Part model, mm, in its own coordinate system. A direction names the side the tool comes from. Coordinates: 2 decimals unless noted, no trailing zeros. Write each loop counter-clockwise with the first axis right and the second up, starting at its lowest first coordinate (ties: lowest second). Pieces come first, ordered by that corner, then holes. Notation, with made-up numbers: (37.5, 29) -> (69.5, 29) arc R31 cw to (69.5, 68) -> close; hole circle Ø11 at (71.25, -27). An arc over 180 degrees is marked (long way). Write item = value, one per line. Start each with the question number.
Q1. Band-saw the part on B-B, the plane x = -5. Give the number of separate pieces and of enclosed holes in the cut face, plus the area to 3 significant figures.
Q2. Band-saw the part on A-A, the plane z = 2.5. List the corners of the cut face in (x, y), plus the area to 3 significant figures.
Q3. Pin check, flat tips, straight feed: P1, Ø1.5, axis at x = -1, y = 4, coming from the +Z side; P2, Ø2, axis at x = -5, y = 5.5, coming from the +Z side; P3, Ø0.8, axis at y = -2, z = 31, coming from the -X side. Stop position of each tip, or through.
Q4. Tool access for faces 5 (the flat face through (-2.724, 6.262, 2.014)), 6 (the flat face through (-1, -1.5, 31)), 7 (the flat face through (-12.365, -1.972, 9.71)): list every direction of +Z, -Z, +X, -X, +Y, -Y with a clear straight run to the whole face (end or side of a thin tool).
Q5. Band-saw the part on C-C, the plane y = 6. List the corners of the cut face in (x, z), plus the area to 3 significant figures.
Q6. Probe line 1 (Z direction, x = -3, y = -3.25); line 2 (X direction, y = 4.75, z = 2); line 3 (Y direction, x = -9.5, z = 19.5). List the from-to ranges inside material, lowest first.
Q7. Pull direction Z, two halves, no side cores. Call faces 1 (the flat face through (-1, 4, 3)), 2 (the flat face through (-1.4, 0, 16.7)), 3 (the flat face through (6.42, -1.97, 21.45)), 4 (the flat face through (18.93, -2, 15)): released by +Z, released by -Z, zero draft, split by the parting line, or undercut.
Q8. Band-saw the part on D-D, the plane x = 1. List the corners of the cut face in (y, z).
from build123d import *

# Parameters (mm, degrees)
F0_W      = 48
F0_H      = 30
F1_DEPTH  = 4
F1_FACE_W = 48
F1_FACE_H = 4
F2_DEPTH  = 1
F3_W      = 40
F3_H      = 1
F4_DEPTH  = 3
F5_W      = 48
F5_H      = 4
F6_DEPTH  = 9
F7_R      = 2
F8_DEPTH  = 4
F9_DEPTH  = 2
F11_DEPTH = 4


with BuildPart() as f1:
    # F0 (on Front) → F1 (new body)
    with BuildSketch(Plane.XZ):
        with Locations((-1.069695, 15)):
            Rectangle(F0_W, F0_H)
        Polygon((-21.069695, 4.268871), (-21.069695, 25.731129), (-3.899889, 15), align=None, mode=Mode.SUBTRACT)
        Polygon((13.700111, 4), (-15.839501, 4), (-1.069695, 13.231129), align=None, mode=Mode.SUBTRACT)
        Polygon((18.930305, 25.731129), (18.930305, 4.268871), (1.760499, 15), align=None, mode=Mode.SUBTRACT)
        Polygon((-1.069695, 16.768871), (-15.839501, 26), (13.700111, 26), align=None, mode=Mode.SUBTRACT)
    extrude(amount=F1_DEPTH)

    # F1_face (on face) → F2 (join)
    with BuildSketch(Plane(origin=(-1.069695, -2, 0), x_dir=(1, 0, 0), z_dir=(0, 0, -1))):
        Rectangle(F1_FACE_W, F1_FACE_H)
    extrude(amount=F2_DEPTH)

    # F3 (on face) → F4 (join)
    with BuildSketch(Plane.XY.offset(30)):
        with Locations((-1.069695, -2)):
            Rectangle(F3_W, F3_H)
    extrude(amount=F4_DEPTH)

    # F5 (on face) → F6 (join)
    with BuildSketch(Plane(origin=(0, 0, 0), x_dir=(-1, 0, 0), z_dir=(0, 1, 0))):
        with Locations((1.069695, 1)):
            Rectangle(F5_W, F5_H)
    extrude(amount=F6_DEPTH)

    # F7 (on face) → F8 (cut)
    with BuildSketch(Plane.XY.offset(3)):
        with Locations((-5.769695, 4.536883)):
            Circle(F7_R)
        with Locations((3.630305, 4.483014)):
            Circle(F7_R)
    extrude(amount=-F8_DEPTH, mode=Mode.SUBTRACT)

    # F7 (on face) → F9 (cut)
    with BuildSketch(Plane.XY.offset(3)):
        Polygon((-3.748969, 1.036883), (-1.728243, 4.536883), (-3.748969, 8.036883), (-7.790421, 8.036883), (-9.811147, 4.536883), (-7.790421, 1.036883), align=None)
        with Locations((-5.769695, 4.536883)):
            Circle(F7_R, mode=Mode.SUBTRACT)
        Polygon((5.651031, 0.983014), (7.671757, 4.483014), (5.651031, 7.983014), (1.609579, 7.983014), (-0.411147, 4.483014), (1.609579, 0.983014), align=None)
        with Locations((3.630305, 4.483014)):
            Circle(F7_R, mode=Mode.SUBTRACT)
    extrude(amount=-F9_DEPTH, mode=Mode.SUBTRACT)

    # F10 (on face) → F11 (cut)
    with BuildSketch(Plane.XY.offset(3)):
        Polygon((-25.069695, 0), (-16.069695, 9), (-25.069695, 9), align=None)
        Polygon((22.930305, 9), (13.930305, 9), (22.930305, 0), align=None)
    extrude(amount=-F11_DEPTH, mode=Mode.SUBTRACT)


solid = f1.part
Ans:
q1.separate_pieces = 5
q1.enclosed_holes = 0
q1.area = 81.9 mm2
q2.outline = (-25.07, -4) -> (22.93, -4) -> (22.93, 0) -> (13.93, 9) -> (-16.07, 9) -> (-25.07, 0) -> close; hole (-9.81, 4.54) -> (-7.79, 1.04) -> (-3.75, 1.04) -> (-1.73, 4.54) -> (-3.75, 8.04) -> (-7.79, 8.04) -> close; hole (-0.41, 4.48) -> (1.61, 0.98) -> (5.65, 0.98) -> (7.67, 4.48) -> (5.65, 7.98) -> (1.61, 7.98) -> close
q2.area = 458 mm2
q3.P1 = 3
q3.P2 = 1
q3.P3 = -21.07
q4.face_5 = +Z
q4.face_6 = +Z, +X, -X, +Y
q4.face_7 = +Y, -Y
q5.outline = (-19.07, -1) -> (-7.13, -1) -> (-7.13, 1) -> (-8.97, 1) -> (-8.97, 3) -> (-19.07, 3) -> close; (-4.41, -1) -> (2.33, -1) -> (2.33, 1) -> (0.46, 1) -> (0.46, 3) -> (-2.57, 3) -> (-2.57, 1) -> (-4.41, 1) -> close; (4.93, -1) -> (16.93, -1) -> (16.93, 3) -> (6.8, 3) -> (6.8, 1) -> (4.93, 1) -> close
q5.area = 108 mm2
q6.line_1 = -1 to 4, 12.02 to 17.98, 26 to 30
q6.line_2 = -20.32 to -9.69, -1.85 to -0.26, 7.52 to 18.18
q6.line_3 = -4 to 0
q7.face_1 = released by +Z
q7.face_2 = zero draft
q7.face_3 = undercut
q7.face_4 = undercut
q8.outline = (-4, -1) -> (9, -1) -> (9, 3) -> (6.93, 3) -> (6.93, 1) -> (2.04, 1) -> (2.04, 3) -> (0, 3) -> (0, 4) -> (-4, 4) -> close; (-4, 11.94) -> (0, 11.94) -> (0, 18.06) -> (-4, 18.06) -> close; (-4, 26) -> (0, 26) -> (0, 30) -> (-1.5, 30) -> (-1.5, 33) -> (-2.5, 33) -> (-2.5, 30) -> (-4, 30) -> close
